from build123d import *

# Parameters (mm, degrees)
SKETCH4_W           = 13.5
SKETCH4_H           = 13.5
SKETCH4_R           = 2.5
HOLE_TOPMAIN_DEPTH  = 64.27
SKETCH12_R          = 2.5
HOLE_SIDE1_DEPTH    = 67.220336
SKETCH13_R          = 3.25
HOLE_SIDE2_DEPTH    = 66.384500568
SKETCH14_R          = 2.5
CUT_EXTRUDE9_DEPTH  = 67.220336097
SKETCH15_R          = 3.25
CUT_EXTRUDE10_DEPTH = 66.384500581
FILLET3_R           = 2
BOSS_EXTRUDE2_START = 20
SKETCH17_R          = 2.5
BOSS_EXTRUDE2_DEPTH = 20


with BuildPart() as part:
    # Sketch4 → hole-TopMain (new body)
    with BuildSketch(Plane(origin=(0, 0, 0), x_dir=(1, 0, 0), z_dir=(0, 1, 0))):
        with Locations((-1.75, 1.75)):
            Rectangle(SKETCH4_W, SKETCH4_H)
        with Locations(Location((0, 0, 0), (0, 0, 90))):
            Circle(SKETCH4_R, mode=Mode.SUBTRACT)
    extrude(amount=HOLE_TOPMAIN_DEPTH)

    # Sketch12 → hole-Side1 (cut, through all)
    with BuildSketch(Plane(origin=(5, 0, 0), x_dir=(0, 0, -1), z_dir=(1, 0, 0))):
        with Locations((1.75, 46.135)):
            Circle(SKETCH12_R)
    extrude(amount=-HOLE_SIDE1_DEPTH, mode=Mode.SUBTRACT)

    # Sketch13 → hole-Side2 (cut, through all)
    with BuildSketch(Plane.ZY.offset(3.5)):
        with Locations((-1.75, 46.135)):
            Circle(SKETCH13_R)
    extrude(amount=-HOLE_SIDE2_DEPTH, mode=Mode.SUBTRACT)

    # Sketch14 → Cut-Extrude9 (cut, through all)
    with BuildSketch(Plane(origin=(0, 0, -8.5), x_dir=(-1, 0, 0), z_dir=(0, 0, -1))):
        with Locations((1.75, 46.135)):
            Circle(SKETCH14_R)
    extrude(amount=-CUT_EXTRUDE9_DEPTH, mode=Mode.SUBTRACT)

    # Sketch15 → Cut-Extrude10 (cut, through all)
    with BuildSketch(Plane(origin=(0, 0, -3.5), x_dir=(-1, 0, 0), z_dir=(0, 0, -1))):
        with Locations((1.75, 46.135)):
            Circle(SKETCH15_R)
    extrude(amount=-CUT_EXTRUDE10_DEPTH, mode=Mode.SUBTRACT)

    # Fillet3
    fillet3_edges = [part.edges().sort_by_distance(p)[0] for p in [
        (-8.5, 32.135, -8.5),
        (-8.5, 32.135, 5),
        (5, 32.135, 5),
        (5, 32.135, -8.5),
    ]]
    fillet(fillet3_edges, radius=FILLET3_R)

    # Sketch17 → Boss-Extrude2 (add)
    with BuildSketch(Plane(origin=(0, 64.27, 0), x_dir=(1, 0, 0), z_dir=(0, 1, 0)).offset(BOSS_EXTRUDE2_START)):
        with BuildLine():
            Line((-8.5, 6.5), (-8.5, -3))
            ThreePointArc((-8.5, -3), (-7.914213562, -4.414213562), (-6.5, -5))
            Line((-6.5, -5), (3, -5))
            ThreePointArc((3, -5), (4.414213562, -4.414213562), (5, -3))
            Line((5, -3), (5, 6.5))
            ThreePointArc((5, 6.5), (4.414213562, 7.914213562), (3, 8.5))
            Line((3, 8.5), (-6.5, 8.5))
            ThreePointArc((-6.5, 8.5), (-7.914213562, 7.914213562), (-8.5, 6.5))
        make_face()
        with Locations(Location((0, 0, 0), (0, 0, 270))):
            Circle(SKETCH17_R, mode=Mode.SUBTRACT)
    extrude(amount=-BOSS_EXTRUDE2_DEPTH)


solid = part.part
Source: CAD feature listing. Evaluate the final solid. Frame: model axes, mm. A direction names the side the tool comes from. Coordinates: 2 decimals unless noted, no trailing zeros. Order: outer loops, then holes, each group sorted by start corner. A loop starts at its lowest first (then second) coordinate and runs counter-clockwise, first axis right, second up.
Item 1: Set-up query: faces 4 (the face through (-4.85, 47.11, 2.58)), 5 (the face through (-2.838, 42.885, -1.776)), 6 (the face through (4.4, 42.72, 4.43)). Return all of +Z, -Z, +X, -X, +Y, -Y with unobstructed straight access to the full face (end or side cutting, diameter ignored); none if empty.
Output values:
face 4: +Z
face 5: +X
face 6: +Z, +X, +Y, -Y
Item 2: Cut plane A-A (y = 13). Return loops of the section in (x, z), plus the area to 3 significant figures.
Output values:
outline: (-8.5, -6.5) arc R2 ccw to (-6.5, -8.5) - (3, -8.5) arc R2 ccw to (5, -6.5) - (5, 3) arc R2 ccw to (3, 5) - (-6.5, 5) arc R2 ccw to (-8.5, 3) - close; hole circle Ø5 at (0, 0)
area: 159 mm2
Item 3: Cut plane B-B (z = -5.75). Return loops of the section in (x, y) (3 decimals).
Output values:
outline: (-8.5, 0) - (5, 0) - (5, 84.27) - (-8.5, 84.27) - close; hole circle Ø5 at (-1.75, 46.135)
Item 4: First-contact query: P1, Ø3, axis at y = 46.135, z = -1.75, coming from the +X side; P2, Ø6, axis at x = -1.75, y = 46.135, coming from the +Z side. Flat tips, straight axial feed; report the tip coordinate or a pass-through.
Output values:
P1: passes through
P2: stops at z = -3.5
Item 5: Cut plane C-C (x = 4). Return loops of the section in (y, z) (3 decimals).
Output values:
outline: (0, -8.232) - (84.27, -8.232) - (84.27, 4.732) - (0, 4.732) - close; hole circle Ø6.5 at (46.135, -1.75)
Item 6: Material intervals for line 1 (X direction, y = 58, z = 0); line 2 (Y direction, x = -1.75, z = -7.4) (3 decimals); line 3 (Z direction, x = -0.25, y = 74), sorted ascending.
Output values:
line 1: x = -8.5 to -2.5, 2.5 to 5
line 2: y = 0 to 43.635, 48.635 to 84.27
line 3: z = -8.5 to -2.49, 2.49 to 5
Item 7: Pull-direction query (Y, two-part tool) for faces 1 (the face through (-1.724, 42.885, -2.838)), 2 (the face through (-2, 0, -2)), 3 (the face through (-2.495, 41.545, -0.165)); classes: pulls with the +Y half, pulls with the -Y half, needs draft (parallel to the pull), parting line crosses it, or undercut.
Output values:
face 1: undercut
face 2: pulls with the -Y half
face 3: needs draft
